from build123d import *

# Parameters (mm, degrees)
F0_W      = 63
F0_H      = 60
F0_W_2    = 53
F0_H_2    = 50
F1_DEPTH  = 20
F3_DEPTH  = 2
F4_DEPTH  = 2
F5_W      = 30
F5_H      = 2
F6_DEPTH  = 1
F7_W      = 30
F7_H      = 2
F8_DEPTH  = 1
F9_R      = 0.99999
F10_W     = 15
F10_H     = 25
F11_DEPTH = 10
F12_W     = 12.5
F12_H     = 20
F13_DEPTH = 8
F14_R     = 2
F15_DEPTH = 25


# Not quite as in the source:
# - a fillet or chamfer is up to 0.001 mm smaller than in the source, because OpenCascade refuses the exact size


with BuildPart() as f1:
    # F0 (on Top) → F1 (new body)
    with BuildSketch(Plane.XY):
        with Locations((19.5141504109, -9.4245311618)):
            Rectangle(F0_W, F0_H)
        with Locations((19.5141504109, -9.4245311618)):
            Rectangle(F0_W_2, F0_H_2, mode=Mode.SUBTRACT)
    extrude(amount=F1_DEPTH)

    # F2 (on Top) → F3 (join)
    with BuildSketch(Plane.XY):
        Polygon((7.0141504109, 25.5754688382), (7.0141504109, 20.5754688382), (9.5141504109, 20.5754688382), (9.5141504109, 23.0754688382), (29.5141504109, 23.0754688382), (29.5141504109, 20.5754688382), (32.0141504109, 20.5754688382), (32.0141504109, 25.5754688382), align=None)
        Polygon((9.5141504109, -39.4245311618), (7.0141504109, -39.4245311618), (7.0141504109, -44.4245311618), (32.0141504109, -44.4245311618), (32.0141504109, -39.4245311618), (29.5141504109, -39.4245311618), (29.5141504109, -41.9245311618), (9.5141504109, -41.9245311618), align=None)
    extrude(amount=F3_DEPTH)

    # F0 (on Top) → F4 (join)
    with BuildSketch(Plane.XY):
        with Locations((19.5141504109, -9.4245311618)):
            Rectangle(F0_W_2, F0_H_2)
    extrude(amount=F4_DEPTH)

    # F5 (on face) → F6 (join)
    with BuildSketch(Plane.XZ.offset(-15.5754688382)):
        with Locations((21.0141504109, 19)):
            Rectangle(F5_W, F5_H)
    extrude(amount=F6_DEPTH)

    # F7 (on face) → F8 (join)
    with BuildSketch(Plane(origin=(0, -34.4245311618, 0), x_dir=(-1, 0, 0), z_dir=(0, 1, 0))):
        with Locations((-18.0141504109, 19)):
            Rectangle(F7_W, F7_H)
    extrude(amount=F8_DEPTH)

    # F9 (radius 1 in the source; OpenCascade refuses exactly that, so slightly less here)
    f9_edges = [f1.edges().sort_by_distance(p)[0] for p in [
        (21.01415, 14.575469, 20),
        (21.01415, 14.575469, 18),
        (18.01415, -33.424531, 20),
        (18.01415, -33.424531, 18),
    ]]
    fillet(f9_edges, radius=F9_R)

    # F10 (on Top) → F11 (join)
    with BuildSketch(Plane.XY):
        with Locations((-19.4858495891, -7.5094338506)):
            Rectangle(F10_W, F10_H)
    extrude(amount=F11_DEPTH)

    # F12 (on face) → F13 (cut)
    with BuildSketch(Plane.XY.offset(10)):
        with Locations((-18.2358495891, -7.5094338506)):
            Rectangle(F12_W, F12_H)
    extrude(amount=-F13_DEPTH, mode=Mode.SUBTRACT)

    # F14 (on face) → F15 (cut)
    with BuildSketch(Plane(origin=(0, 4.9905661494, 0), x_dir=(-1, 0, 0), z_dir=(0, 1, 0))):
        with Locations((19.4858495891, 6.5377363935)):
            Circle(F14_R)
    extrude(amount=-F15_DEPTH, mode=Mode.SUBTRACT)


solid = f1.part
Verification items for the finished model (mm, model axes). A direction names the side the tool comes from. Give positions to 0.01 mm unless a question says otherwise; leave off trailing zeros. Write each loop counter-clockwise with the first axis right and the second up, starting at its lowest first coordinate (ties: lowest second). Pieces come first, ordered by that corner, then holes. Notation, with made-up numbers: M -13,11 L 14,11 A27 ccw 14,34 Z; hole C 70.25,43.25 d10. An arc over 180 degrees is marked long. Use CSV: the item, a comma, the result in double quotes.
1) Release check for a two-part mould opening along X. For faces 1 (the face through (-20, 4.991, 4)), 2 (the face through (32.014, -42, 1)), 3 (the face through (29.514, 22, 1)) record: released by +X, released by -X, zero draft, split by the parting line, or undercut.
Final values:
face 1,"zero draft"
face 2,"released by +X"
face 3,"undercut"
2) Access from +Z, -Z, +X, -X, +Y, -Y to the whole of each face (thin tool, end or side, straight path). Record for faces 4 (the face through (-20, -20.009, 4)), 5 (the face through (19, -43, 2)), 6 (the face through (9.514, -41, 1)), 7 (the face through (46.014, -10, 11)).
Final values:
face 4,"+Z, -Z, -X, -Y"
face 5,"+Z, +X, -X, -Y"
face 6,"+Z, -Z"
face 7,"+Z"
3) Material ranges on line 1 along X through (y, z) = (-5, 6.5); line 2 along X through (y, z) = (3, 16.75); line 3 along Y through (x, z) = (39, 10.5), recorded low to high.
Final values:
line 1,"-26.99 to -24.49, -11.99 to -6.99, 46.01 to 51.01"
line 2,"-11.99 to -6.99, 46.01 to 51.01"
line 3,"-39.42 to -34.42, 15.58 to 20.58"
4) Cross-section at D-D (y = -27). Enter the section's corners in (x, z).
Final values:
outline,"M -11.99,0 L 51.01,0 L 51.01,20 L 46.01,20 L 46.01,2 L -6.99,2 L -6.99,20 L -11.99,20 Z"
5) Cross-section at B-B (z = 13.25). Enter the section's corners in (x, y).
Final values:
outline,"M -11.99,-39.42 L 51.01,-39.42 L 51.01,20.58 L -11.99,20.58 Z; hole M -6.99,-34.42 L 46.01,-34.42 L 46.01,15.58 L -6.99,15.58 Z"
6) Cross-section at C-C (y = 4). Enter the section's corners in (x, z), plus the area to 3 significant figures.
Final values:
outline,"M -26.99,0 L 51.01,0 L 51.01,20 L 46.01,20 L 46.01,2 L -6.99,2 L -6.99,20 L -11.99,20 L -11.99,10 L -26.99,10 Z; hole C -19.49,6.54 d4"
area,"443 mm²"
7) Go/stop test with flat-tipped pins: pin 1 Ø6 at (x, y) = (-16, -8.5) entering from +Z; pin 2 Ø1 at (y, z) = (-40.5, 1.5) entering from +X; pin 3 Ø10 at (x, z) = (17.5, 16.5) entering from -Y; pin 4 Ø5 at (y, z) = (-8, 11) entering from -X. Record where each tip stops, or that it passes through.
Final values:
pin 1,"z = 2"
pin 2,"x = 32.01"
pin 3,"y = -39.42"
pin 4,"x = -26.99"
8) Cross-section at A-A (x = 21). State how many separate pieces and enclosed holes the cut face has, plus the area to 3 significant figures.
Final values:
separate pieces,"3"
enclosed holes,"0"
area,"313 mm²"
